Work out the finished part from the listing and answer in its coordinate system (mm). Face numbers are marked on the shaded views. A direction names the side the tool comes from. Round coordinates to 2 decimals unless told otherwise and drop trailing zeros. Order: outer loops, then holes, each group sorted by start corner. A loop starts at its lowest first (then second) coordinate and runs counter-clockwise, first axis right, second up. Notation, with made-up numbers: (-9, 3) - (49, 3) arc R29 ccw to (49, 35) - close; hole circle Ø7 at (-20.5, 56.25). An arc over 180 degrees is marked (long way). Put each result on its own line as item: value.
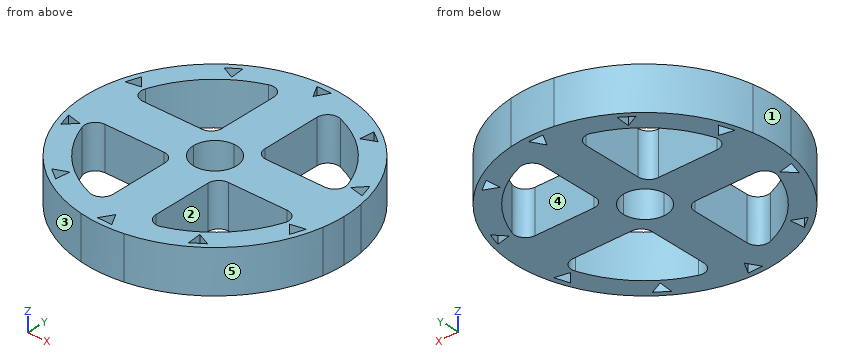
```python
from build123d import *

# Parameters (mm, degrees)
F1_DEPTH = 12.7


with BuildPart() as f1:
    # F0 (on Top) → F1 (new body, symmetric)
    with BuildSketch(Plane.XY):
        with BuildLine():
            ThreePointArc((75.134213, -12.7), (75.933086, -6.372321), (76.2, 0))
            ThreePointArc((76.2, 0), (75.933086, 6.372321), (75.134213, 12.7))
            ThreePointArc((75.134213, 12.7), (53.881537, 53.881537), (12.7, 75.134213))
            ThreePointArc((12.7, 75.134213), (0, 76.2), (-12.7, 75.134213))
            ThreePointArc((-12.7, 75.134213), (-53.881537, 53.881537), (-75.134213, 12.7))
            ThreePointArc((-75.134213, 12.7), (-76.2, 0), (-75.134213, -12.7))
            ThreePointArc((-75.134213, -12.7), (-53.881537, -53.881537), (-12.7, -75.134213))
            ThreePointArc((-12.7, -75.134213), (0, -76.2), (12.7, -75.134213))
            ThreePointArc((12.7, -75.134213), (53.881537, -53.881537), (75.134213, -12.7))
        make_face()
        Polygon((-39.219381, -52.680772), (-40.204984, -61.113142), (-47.01483, -56.0434), align=None, mode=Mode.SUBTRACT)
        Polygon((-0.636809, -65.673572), (3.53659, -73.066746), (-4.952786, -72.984428), align=None, mode=Mode.SUBTRACT)
        Polygon((-62.731954, -19.445449), (-68.497842, -25.676887), (-71.011482, -17.567763), align=None, mode=Mode.SUBTRACT)
        with BuildLine():
            ThreePointArc((-21.166667, -59.868374), (-44.901281, -44.901281), (-59.868374, -21.166667))
            ThreePointArc((-59.868374, -21.166667), (-59.06629, -15.383826), (-53.881537, -12.7))
            Line((-53.881537, -12.7), (-19.05, -12.7))
            ThreePointArc((-19.05, -12.7), (-14.559872, -14.559872), (-12.7, -19.05))
            Line((-12.7, -19.05), (-12.7, -53.881537))
            ThreePointArc((-12.7, -53.881537), (-15.383826, -59.06629), (-21.166667, -59.868374))
        make_face(mode=Mode.SUBTRACT)
        Polygon((38.190457, -53.431382), (45.919233, -56.944542), (39.012359, -61.881279), align=None, mode=Mode.SUBTRACT)
        with BuildLine():
            ThreePointArc((12.7, -19.05), (14.559872, -14.559872), (19.05, -12.7))
            Line((19.05, -12.7), (53.881537, -12.7))
            ThreePointArc((53.881537, -12.7), (59.06629, -15.383826), (59.868374, -21.166667))
            ThreePointArc((59.868374, -21.166667), (44.901281, -44.901281), (21.166667, -59.868374))
            ThreePointArc((21.166667, -59.868374), (15.383826, -59.06629), (12.7, -53.881537))
            Line((12.7, -53.881537), (12.7, -19.05))
        make_face(mode=Mode.SUBTRACT)
        Polygon((62.343086, -20.658249), (70.657467, -18.941467), (67.987053, -27.000324), align=None, mode=Mode.SUBTRACT)
        Polygon((-62.13985, 21.261764), (-70.470487, 19.62568), (-67.722059, 27.658265), align=None, mode=Mode.SUBTRACT)
        with BuildLine():
            Line((-12.7, 53.881537), (-12.7, 19.05))
            ThreePointArc((-12.7, 19.05), (-14.559872, 14.559872), (-19.05, 12.7))
            Line((-19.05, 12.7), (-53.881537, 12.7))
            ThreePointArc((-53.881537, 12.7), (-59.06629, 15.383826), (-59.868374, 21.166667))
            ThreePointArc((-59.868374, 21.166667), (-44.901281, 44.901281), (-21.166667, 59.868374))
            ThreePointArc((-21.166667, 59.868374), (-15.383826, 59.06629), (-12.7, 53.881537))
        make_face(mode=Mode.SUBTRACT)
        Polygon((-37.670584, 53.79917), (-45.364933, 57.387104), (-38.410517, 62.256639), align=None, mode=Mode.SUBTRACT)
        with BuildLine():
            ThreePointArc((0, 12.7), (8.980256, 8.980256), (12.7, 0))
            ThreePointArc((12.7, 0), (8.980256, -8.980256), (0, -12.7))
            ThreePointArc((0, -12.7), (-8.980256, -8.980256), (-12.7, 0))
            ThreePointArc((-12.7, 0), (-8.980256, 8.980256), (0, 12.7))
        make_face(mode=Mode.SUBTRACT)
        with BuildLine():
            ThreePointArc((19.05, 12.7), (14.559872, 14.559872), (12.7, 19.05))
            Line((12.7, 19.05), (12.7, 53.881537))
            ThreePointArc((12.7, 53.881537), (15.383826, 59.06629), (21.166667, 59.868374))
            ThreePointArc((21.166667, 59.868374), (44.901281, 44.901281), (59.868374, 21.166667))
            ThreePointArc((59.868374, 21.166667), (59.06629, 15.383826), (53.881537, 12.7))
            Line((53.881537, 12.7), (19.05, 12.7))
        make_face(mode=Mode.SUBTRACT)
        Polygon((62.54046, 20.052792), (68.245656, 26.339844), (70.837805, 18.255473), align=None, mode=Mode.SUBTRACT)
        Polygon((-4.244888, 73.02902), (4.244888, 73.02902), (0, 65.676659), align=None, mode=Mode.SUBTRACT)
        Polygon((38.706739, 53.058571), (39.610534, 61.500102), (46.469216, 56.496627), align=None, mode=Mode.SUBTRACT)
    extrude(amount=F1_DEPTH, both=True)


solid = f1.part
```
1) A cutting plane is placed at A-A on x = -8.5. Write down the section's boundary in (y, z).
Findings below:
outline: (-75.72, -12.7) - (-9.44, -12.7) - (-9.44, 12.7) - (-75.72, 12.7) - close; (9.44, -12.7) - (75.72, -12.7) - (75.72, 12.7) - (9.44, 12.7) - close
2) For a pull along X with two mould halves and no side action, classify the marked faces 3, 4 and 5 as pulls with the +X half, pulls with the -X half, needs draft (parallel to the pull), parting line crosses it, or undercut.
Findings below:
face 3: pulls with the -X half
face 4: undercut
face 5: pulls with the +X half
3) A cutting plane is placed at C-C on x = 48.5. Write down the section's boundary in (y, z).
Findings below:
outline: (-58.77, -12.7) - (-40.99, -12.7) - (-40.99, 12.7) - (-58.77, 12.7) - close; (-12.7, -12.7) - (12.7, -12.7) - (12.7, 12.7) - (-12.7, 12.7) - close; (40.99, -12.7) - (58.77, -12.7) - (58.77, 12.7) - (40.99, 12.7) - close
4) A cutting plane is placed at D-D on x = -42.5. Write down the section's boundary in (y, z), then the cut area to 3 significant figures.
Findings below:
outline: (-63.25, -12.7) - (-59.4, -12.7) - (-59.4, 12.7) - (-63.25, 12.7) - close; (-54.1, -12.7) - (-47.18, -12.7) - (-47.18, 12.7) - (-54.1, 12.7) - close; (-12.7, -12.7) - (12.7, -12.7) - (12.7, 12.7) - (-12.7, 12.7) - close; (47.18, -12.7) - (56.05, -12.7) - (56.05, 12.7) - (47.18, 12.7) - close; (59.39, -12.7) - (63.25, -12.7) - (63.25, 12.7) - (59.39, 12.7) - close
area: 1,240 mm2
5) For the marked faces 1 and 2, determine the directions among +Z, -Z, +X, -X, +Y, -Y from which every point of the face is accessible in a straight line to the end or side of a thin tool.
Findings below:
face 1: +Z, -Z, -X
face 2: +Z, -Z
6) Straight lines are drawn through the part: L1, parallel to Y at x = 23, z = 7.5; L2, parallel to X at y = 37.5, z = 2; L3, parallel to X at y = 23, z = 9.75. For each, find the intervals that lie inside material, in ascending order. Write a range as from..to.
Findings below:
L1: y = -72.65..-59.19, -12.7..12.7, 59.19..72.65
L2: x = -66.33..-51.24, -12.7..12.7, 51.24..66.33
L3: x = -72.65..-69.32, -63.66..-59.19, -12.7..12.7, 59.19..65.21, 69.32..72.65
7) A cutting plane is placed at B-B on y = 43.5. Write down the section's boundary in (x, z).
Findings below:
outline: (-62.56, -12.7) - (-46.26, -12.7) - (-46.26, 12.7) - (-62.56, 12.7) - close; (-12.7, -12.7) - (12.7, -12.7) - (12.7, 12.7) - (-12.7, 12.7) - close; (46.26, -12.7) - (62.56, -12.7) - (62.56, 12.7) - (46.26, 12.7) - close
8) Given pin 1 Ø4 at (x, z) = (49.5, -3.5) entering from +Y; pin 2 Ø7.5 at (x, z) = (-40.5, -3) entering from -Y; pin 3 Ø12 at (x, y) = (23.5, -42.5) entering from -Z; pin 4 Ø1.5 at (y, z) = (-24.5, 5.5) entering from -X, each flat-ended and moving along its own axis, determine where each tip first touches the part or whether it passes through.
Findings below:
pin 1: stops at y = 59.58
pin 2: stops at y = -66.75
pin 3: passes through
pin 4: stops at x = -72.4
